Answer from the drawing. Dimensions are ordinates in mm from the lowest x, y and z of the part. Coordinates: 2 decimals unless noted, no trailing zeros. Write each loop counter-clockwise with the first axis right and the second up, starting at its lowest first coordinate (ties: lowest second). Pieces come first, ordered by that corner, then holes.
1) Find the intervals of material crossed by line 1 (Z direction, x = 10, y = 11.5); line 2 (Y direction, x = 14, z = 9); line 3 (X direction, y = 12.25, z = 11), in increasing order.
2) Each of these flat-tipped pins is pushed along its axis until it touches: pin 1 Ø4 at (x, z) = (10, 10) entering from +Y; pin 2 Ø4 at (x, y) = (8, 18.5) entering from -Z; pin 3 Ø5 at (x, z) = (16.5, 9.5) entering from -Y; pin 4 Ø1.5 at (x, y) = (15, 7) entering from +Z. Where does it stop, or does it pass through?
3) Determine the mould class of the marked faces 1, 2 and 3 for opening direction X: +X half, -X half, draft (parallel to the pull), parting line (faces both ways), or undercut.
4) The part is cut by section A-A (x = 10). Determine the outline of the cut face in (y, z).
5) The part is cut by section B-B (y = 2). Determine the outline of the cut face in (x, z), then the cut area to 3 significant figures.
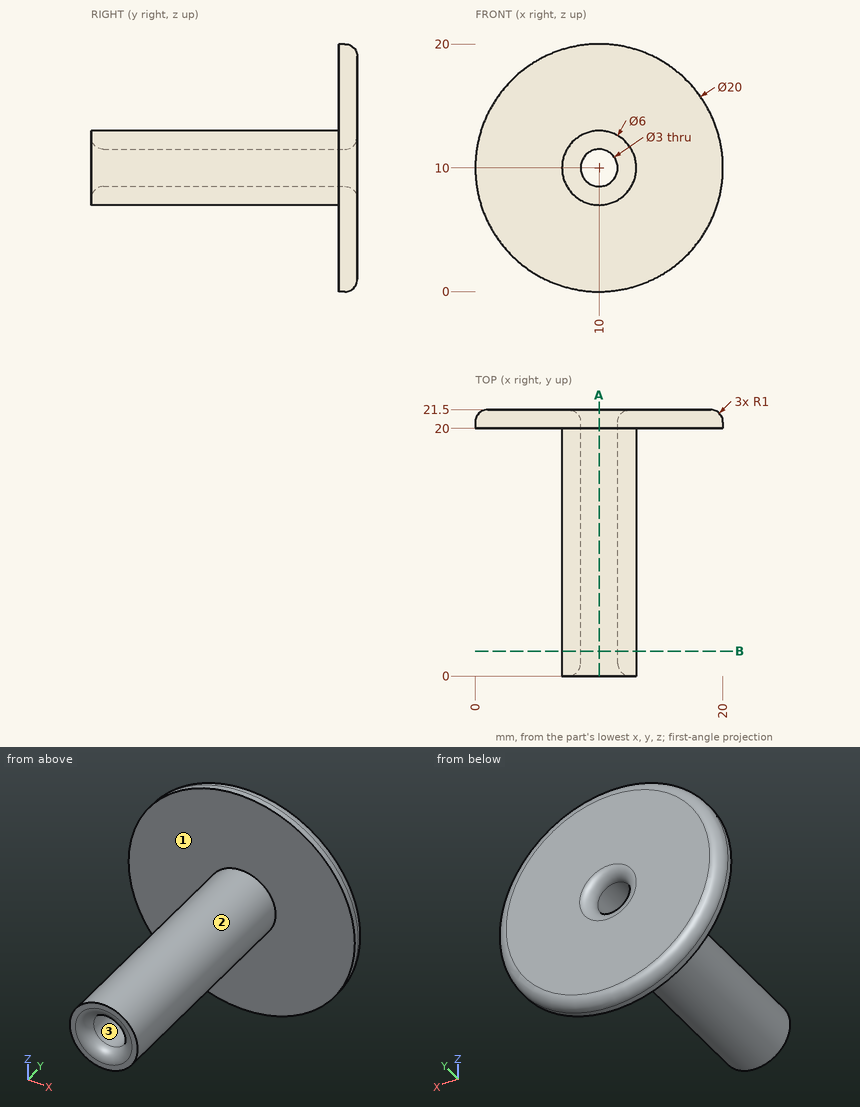
Reported:
1. line 1: z = 7 to 8.5, 11.5 to 13
1. line 2: y = 20 to 21.5
1. line 3: x = 7.17 to 8.88, 11.12 to 12.83
2. pin 1: stops at y = 21.37
2. pin 2: stops at z = 0.02
2. pin 3: stops at y = 20
2. pin 4: passes through
3. face 1: draft
3. face 2: parting line
3. face 3: undercut
4. outline: (0, 7) - (20, 7) - (20, 0) - (20.5, 0) arc R1 ccw to (21.5, 1) - (21.5, 7.5) arc R1 ccw to (20.5, 8.5) - (1, 8.5) arc R1 ccw to (0, 7.5) - close; (0, 12.5) arc R1 ccw to (1, 11.5) - (20.5, 11.5) arc R1 ccw to (21.5, 12.5) - (21.5, 19) arc R1 ccw to (20.5, 20) - (20, 20) - (20, 13) - (0, 13) - close
5. outline: circle Ø6 at (10, 10); hole circle Ø3 at (10, 10)
5. area: 21.2 mm2
